```python
from build123d import *

# Parameters (mm, degrees)
AUFSATZ_LINEAR_AUSTRAGEN1_DEPTH = 10
VERRUNDUNG11_R                  = 15
VERRUNDUNG12_R                  = 5
VERRUNDUNG13_R                  = 3
VERRUNDUNG14_R                  = 3
WANDUNG1_T                      = -2


with BuildPart() as part:
    # Skizze1 → Aufsatz-Linear austragen1 (new body)
    with BuildSketch(Plane(origin=(0, 0, 0), x_dir=(1, 0, 0), z_dir=(0, 1, 0))):
        Polygon((0, -75.745036748), (-24.999786643, -75.641751751), (-37.792132404, -60.267881388), (-37.855752194, 24.732118612), (-25, 40.053007474), (0, 40.053007474), align=None)
    aufsatz_linear_austragen1 = extrude(amount=AUFSATZ_LINEAR_AUSTRAGEN1_DEPTH)

    # Spiegeln1: Aufsatz-Linear austragen1 across plane
    add(aufsatz_linear_austragen1.mirror(Plane(origin=(0, 0, 0), x_dir=(0, 0, 1), z_dir=(1, 0, 0))))

    # Verrundung11
    verrundung11_edges = [part.edges().sort_by_distance(p)[0] for p in [
        (-24.999786643, 5, 75.641751751),
        (24.999786643, 5, 75.641751751),
    ]]
    fillet(verrundung11_edges, radius=VERRUNDUNG11_R)

    # Verrundung12
    verrundung12_edges = [part.edges().sort_by_distance(p)[0] for p in [
        (-37.792132404, 5, 60.267881388),
        (37.792132404, 5, 60.267881388),
    ]]
    fillet(verrundung12_edges, radius=VERRUNDUNG12_R)

    # Verrundung13
    verrundung13_edges = [part.edges().sort_by_distance(p)[0] for p in [
        (-25, 5, -40.053007474),
        (25, 5, -40.053007474),
    ]]
    fillet(verrundung13_edges, radius=VERRUNDUNG13_R)

    # Verrundung14
    verrundung14_edges = [part.edges().sort_by_distance(p)[0] for p in [
        (-37.855752194, 5, -24.732118612),
        (37.855752194, 5, -24.732118612),
    ]]
    fillet(verrundung14_edges, radius=VERRUNDUNG14_R)

    # Wandung1
    wandung1_openings = [part.faces().sort_by_distance(p)[0] for p in [
        (0, 10, 17.703317915),
    ]]
    offset(amount=WANDUNG1_T, openings=wandung1_openings, kind=Kind.INTERSECTION)


solid = part.part
```
For this review, take the finished solid that the model builds, in its own axes (mm). A direction names the side the tool comes from. Give positions to 0.01 mm unless a question says otherwise; leave off trailing zeros. Write each loop counter-clockwise with the first axis right and the second up, starting at its lowest first coordinate (ties: lowest second). Pieces come first, ordered by that corner, then holes. Notation, with made-up numbers: M 48.5,-4.75 L 63.5,-4.75 A19 cw 63.5,9.25 Z; hole C 83,64 d2. An arc over 180 degrees is marked long. One line per item, written item: value.
1) For line 1 (Z direction, x = -17, y = 4); line 2 (X direction, y = 2.5, z = -15), list the stretches that pass through material, from the lowest coordinate up. Write a range as from..to.
Results are:
line 1: z = -40.05..-38.05, 73.67..75.67
line 2: x = -37.85..-35.85, 35.85..37.85
2) Take a section at B-B, the plane z = 39.5. Write out the cut boundary in (x, y), then the cut area to 3 significant figures.
Results are:
outline: M -37.81,0 L 37.81,0 L 37.81,10 L 35.81,10 L 35.81,2 L -35.81,2 L -35.81,10 L -37.81,10 Z
area: 183 mm²
3) The part is to be moulded in two halves that separate along Z. For faces 1 (the flat face through (36, 10, 5)), 2 (the cylindrical face through (37.487, 5.07, 60.183)), 3 (the cylindrical face through (23.414, 6.056, 72.464)), say which applies: +Z half, -Z half, draft (parallel to the pull), parting line (faces both ways), or undercut.
Results are:
face 1: draft
face 2: +Z half
face 3: undercut
4) Take a section at C-C, the plane x = 33.5. Write out the cut boundary in (y, z), then the cut area to 3 significant figures.
Results are:
outline: M 0,-29.92 L 10,-29.92 L 10,-26.81 L 2,-26.81 L 2,62.3 L 10,62.3 L 10,65.43 L 0,65.43 Z
area: 241 mm²
5) For P1, Ø1.5, axis at x = 11.5, z = 15, coming from the +Y side; P2, Ø6, axis at y = 6.5, z = 7, coming from the -X side; P3, Ø2.5, axis at x = 8, y = 6.5, coming from the +Z side, all flat-tipped, find the tip position at first contact; note any pin that passes through.
Results are:
P1: stops at y = 2
P2: stops at x = -37.83
P3: stops at z = 75.72
6) For faces 4 (the cylindrical face through (-23.558, 6.056, 72.396)), 5 (the flat face through (-1, 0, 17)), list the 3-axis set-ups (+Z, -Z, +X, -X, +Y, -Y) from which the entire face can be reached by the end or side of a thin tool; tool diameter is ignored.
Results are:
face 4: +Y
face 5: +Z, -Z, +X, -X, -Y
